Autodesk Inventor part; units mm, degrees
ref_plane "YZ Plane" through (0, 0, 0) normal (1, 0, 0) x (0, 1, 0)
ref_plane "XZ Plane" through (0, 0, 0) normal (0, 1, 0) x (-1, 0, 0)
ref_plane "XY Plane" through (0, 0, 0) normal (0, 0, 1) x (1, 0, 0)
sketch "Sketch1" plane through (0, 0, 0) normal (0, 0, 1) x (1, 0, 0)
  circle A0 centre (0, 0) radius 17.5
  dimension "d0" = 35
extrude "Extrusion1" add sketch "Sketch1" along normal blind 5
sketch "Sketch2" plane through (0, 0, 5) normal (0, 0, 1) x (1, 0, 0)
  line L0 (-19, -50) -> (19, -50)
  line L1 (19, -50) -> (19, 50)
  line L2 (19, 50) -> (-19, 50)
  line L3 (-19, 50) -> (-19, -50)
  line L4 (-19, -50) -> (19, 50) construction
  line L5 (19, -50) -> (-19, 50) construction
  point P0 (0, 0)
  dimension "d3" = 38
  dimension "d4" = 100
extrude "Extrusion2" add sketch "Sketch2" along normal blind 8
sketch "Sketch3" plane through (0, 0, 13) normal (0, 0, 1) x (1, 0, 0)
  point P0 (0, 0)
  point P1 (14, 0)
  dimension "d7" = 14
hole "Hole1" at (14, 0, 13) direction (0, 0, -1) diameter 3.4 end through all counterbore diameter 6.5 counterbore depth 4
pattern_circular "Circular Pattern1" count 6 over 360 about axis through (0, 0, -10) along (0, 0, 1) of "Hole1"
sketch "Sketch4" plane through (0, 0, 5) normal (0, 0, -1) x (-1, 0, 0)
  line L0 (-16, 45) -> (16, 45)
  line L1 (16, 45) -> (16, 35)
  line L2 (16, 35) -> (-16, 35)
  line L3 (-16, 35) -> (-16, 45)
  line L4 (-16, 45) -> (16, 35) construction
  line L5 (16, 45) -> (-16, 35) construction
  line L6 (-19, 50) -> (19, 50)
  line L7 (19, 50) -> (19, -50)
  line L8 (-19, -50) -> (-19, 50)
  point P0 (0, 0)
  point P1 (0, 40)
  dimension "d18" = 5
  dimension "d19" = 3
  dimension "d20" = 3
  dimension "d21" = 10
hole "Hole2" at (16, 45, 5) at (-16, 45, 5) at (-16, 35, 5) at (16, 35, 5) direction (0, 0, 1) diameter 3.4 end through all counterbore diameter 6.5 counterbore depth 3.4
mirror "Mirror1" about plane through (0, 0, 0) normal (0, 1, 0) of "Hole2"
fillet "Fillet1" radius 2 1 edges at (-17.5, 0, 5)
fillet "Fillet2" radius 1 16 edges at (-19, -33.75, 6.7) (-19, -36.25, 6.7) (-19, -43.75, 6.7) (-19, -46.25, 6.7) (19, -33.75, 6.7) (19, -36.25, 6.7) (19, -43.75, 6.7) (19, -46.25, 6.7) (19, 33.75, 6.7) (19, 36.25, 6.7) (19, 43.75, 6.7) (19, 46.25, 6.7) (-19, 33.75, 6.7) (-19, 36.25, 6.7) (-19, 43.75, 6.7) (-19, 46.25, 6.7)
ref_plane "Work Plane1" through (0, 0, 0) normal (0, 1, 0) x (-1, 0, 0)
equation "\"d19\" = d20"
equation "\"d21\" = 2 * d18"
properties part number "401-flange"
Part model, mm, in its own coordinate system. A direction names the side the tool comes from. Give positions to 0.01 mm unless a question says otherwise; leave off trailing zeros. Write each loop counter-clockwise with the first axis right and the second up, starting at its lowest first coordinate (ties: lowest second). Pieces come first, ordered by that corner, then holes.
1) Cut at A-A on y = 45. Write the cut outline in (x, z).
Resolved:
outline: (-19, 8.4) - (-17.7, 8.4) - (-17.7, 13) - (-19, 13) - close; (-14.3, 8.4) - (-12.75, 8.4) - (-12.75, 5) - (12.75, 5) - (12.75, 8.4) - (14.3, 8.4) - (14.3, 13) - (-14.3, 13) - close; (17.7, 8.4) - (19, 8.4) - (19, 13) - (17.7, 13) - close
2) Which spindle directions (+Z, -Z, +X, -X, +Y, -Y) get a long thin tool onto all of the face, cutting with end or side? Do faces 4 (the face through (17.03, 33.65, 10.73)), 5 (the face through (9, 13, 9)), 6 (the face through (12.75, -34.91, 6.72)). Say none if no direction does.
Resolved:
face 4: +Z, -Z
face 5: +Z
face 6: -Z
3) Cut at D-D on y = 28. Write the cut outline in (x, z), then the cut area to 3 significant figures.
Resolved:
outline: (-19, 5) - (19, 5) - (19, 13) - (-19, 13) - close
area: 304 mm2
4) Probe L1, parallel to Y at x = -16, z = 10.4; L2, parallel to X at y = 42, z = 7; L3, parallel to Y at x = 16, z = 7. List the from-to ranges inside material, lowest first.
Resolved:
L1: y = -50 to -46.7, -43.3 to -36.7, -33.3 to -2.56, 2.56 to 33.3, 36.7 to 43.3, 46.7 to 50
L2: x = -18.66 to -17.25, -14.75 to 14.75, 17.25 to 18.66
L3: y = -50 to -48.25, -41.75 to -38.25, -31.75 to 31.75, 38.25 to 41.75, 48.25 to 50
5) Two-plate mould, pull along Y, no slides. Class faces 1 (the face through (0, 50, 9)), 2 (the face through (0, 0, 0)), 3 (the face through (-12.75, 44.91, 6.72)): released by +Y, released by -Y, zero draft, split by the parting line, or undercut.
Resolved:
face 1: released by +Y
face 2: zero draft
face 3: undercut
6) Cut at B-B on x = 0. Write the cut outline in (y, z).
Resolved:
outline: (-50, 5) - (-19.5, 5) arc R2 cw to (-17.5, 3) - (-17.5, 0) - (17.5, 0) - (17.5, 3) arc R2 cw to (19.5, 5) - (50, 5) - (50, 13) - (-50, 13) - close
7) Pin check, flat tips, straight feed: pin 1 (1.9 mm diameter, centred on x = -16, y = -33.5, fed in from -Z); pin 2 (4.5 mm diameter, centred on x = 14, y = 0, fed in from -Z); pin 3 (3 mm diameter, centred on x = -15.5, y = 47, fed in from -Z). Stop position of each tip, or through.
Resolved:
pin 1: stops at z = 8.4
pin 2: stops at z = 0
pin 3: stops at z = 5
8) Cut at C-C on z = 1.25. Write the cut outline in (x, y).
Resolved:
outline: circle Ø35 at (0, 0); hole circle Ø3.4 at (-14, 0); hole circle Ø3.4 at (-7, -12.12); hole circle Ø3.4 at (-7, 12.12); hole circle Ø3.4 at (7, -12.12); hole circle Ø3.4 at (7, 12.12); hole circle Ø3.4 at (14, 0)
